Check sheet for the modelled part. Datum: model origin and axes. Units: mm. A direction names the side the tool comes from. Round coordinates to 2 decimals unless told otherwise and drop trailing zeros. Order: outer loops, then holes, each group sorted by start corner. A loop starts at its lowest first (then second) coordinate and runs counter-clockwise, first axis right, second up.
Q1. Scan lines: probe 1 along Z at (x, y) = (1.5, 13); probe 2 along X at (y, z) = (112, -3.75); probe 3 along Y at (x, z) = (0.5, -3). Record each from-to range of solid material in increasing order.
Q2. Depth check by flat-ended pin: P1, Ø5, axis at y = 178, z = 2, coming from the +X side; P2, Ø8, axis at x = -4, z = 6, coming from the +Y side; P3, Ø3, axis at y = 23, z = -1, coming from the +X side; P4, Ø3, axis at x = 7.5, y = 148.5, coming from the +Z side. Enter the tip coordinate at first touch or a pass-through.
Q3. Set-up check for faces 1 (the cylindrical face through (2.44, 49.3, 0.54)), 2 (the flat face through (0, 200, 0)): record each of +Z, -Z, +X, -X, +Y, -Y from which the full face is reachable in a straight line by a thin tool's end or side.
Q4. Cross-section at A-A on y = 33. Record the cut outline in (x, z).
from build123d import *

# Parameters (mm, degrees)
SKETCH1_R           = 2.5
BOSS_EXTRUDE1_DEPTH = 100
SKETCH3_R           = 10
SKETCH2_R           = 5
FILLET1_R           = 5


with BuildPart() as part:
    # Sketch1 → Boss-Extrude1 (new body)
    with BuildSketch(Plane(origin=(0, 0, 0), x_dir=(1, 0, 0), z_dir=(0, 1, 0))):
        with Locations(Location((0, 0, 0), (0, 0, 90))):
            Circle(SKETCH1_R)
    extrude(amount=BOSS_EXTRUDE1_DEPTH)

    # Sketch3 → Loft1 section 0
    with BuildSketch(Plane(origin=(0, 200, 0), x_dir=(1, 0, 0), z_dir=(0, 1, 0))):
        Circle(SKETCH3_R)
    # Sketch2 → Loft1 section 1
    with BuildSketch(Plane(origin=(0, 100, 0), x_dir=(1, 0, 0), z_dir=(0, 1, 0))):
        Circle(SKETCH2_R)
    loft()

    # Fillet1
    # the kernel refuses this fillet: 5 mm, written as the material it takes off along each edge
    with BuildSketch(Plane(origin=(0, 200, 0), x_dir=(1, 0, 0), z_dir=(0, 0, 1))) as fillet1_piece_1:
        with BuildLine():
            CenterArc((10 - FILLET1_R * 1.05124921973, -FILLET1_R), FILLET1_R, 357.137594774, 92.862405226)
            Line((10 - FILLET1_R * 1.05124921973, 0), (10 - FILLET1_R * 1.05124921973, FILLET1_R * 0.02))
            Line((10 - FILLET1_R * 1.05124921973, FILLET1_R * 0.02), (10 + FILLET1_R * 0.0210249843945, FILLET1_R * 0.02))
            Line((10 + FILLET1_R * 0.0210249843945, FILLET1_R * 0.02), (10 - FILLET1_R * 0.0325218340696, -FILLET1_R * 1.05093636928))
            Line((10 - FILLET1_R * 0.0325218340696, -FILLET1_R * 1.05093636928), (10 - FILLET1_R * 0.0524968808472, -FILLET1_R * 1.04993761694))
        make_face()
    revolve(axis=Axis((0, 200, 0), (0, 1, 0)), mode=Mode.SUBTRACT)
    with BuildSketch(Plane(origin=(0, 100, 0), x_dir=(1, 0, 0), z_dir=(0, 0, 1))) as fillet1_piece_2:
        with BuildLine():
            CenterArc((0.216150111, 4.4479242), FILLET1_R, 297.178875661, 59.958719113)
            Line((2.5, 0), (2.545676998, -0.088958484))
            ThreePointArc((2.545676998, -0.088958484), (3.75, -0.1), (5, -0.1))
            Line((5, -0.1), (5.099875234, -0.004993762))
            Line((5.099875234, -0.004993762), (5.30978704, 4.193242353))
            Line((5.30978704, 4.193242353), (5.209911806, 4.198236115))
        make_face()
    revolve(axis=Axis((0, 100, 0), (0, 1, 0)), mode=Mode.SUBTRACT)


solid = part.part
Results found:
1. probe 1: z = -2 to 2
1. probe 2: x = -4.16 to 4.16
1. probe 3: y = 100.32 to 200
2. P1: stops at x = 8.99
2. P2: stops at y = 200
2. P3: stops at x = 2.5
2. P4: stops at z = 4.38
3. face 1: -Y
3. face 2: +Z, -Z, +X, -X, +Y
4. outline: circle Ø5 at (0, 0)
